Could you check a few things on this drawing? It's one solid part, dimensions in mm from its lowest x, y, z. Give positions to 0.01 mm unless a question says otherwise; leave off trailing zeros. Order: outer loops, then holes, each group sorted by start corner. A loop starts at its lowest first (then second) coordinate and runs counter-clockwise, first axis right, second up. Notation, with made-up numbers: M 11.5,-20.75 L 60.5,-20.75 A24 ccw 60.5,-6.75 Z; hole C 62,54.25 d2. An arc over 180 degrees is marked long. One line per item, written item: value. Start each with the question number.
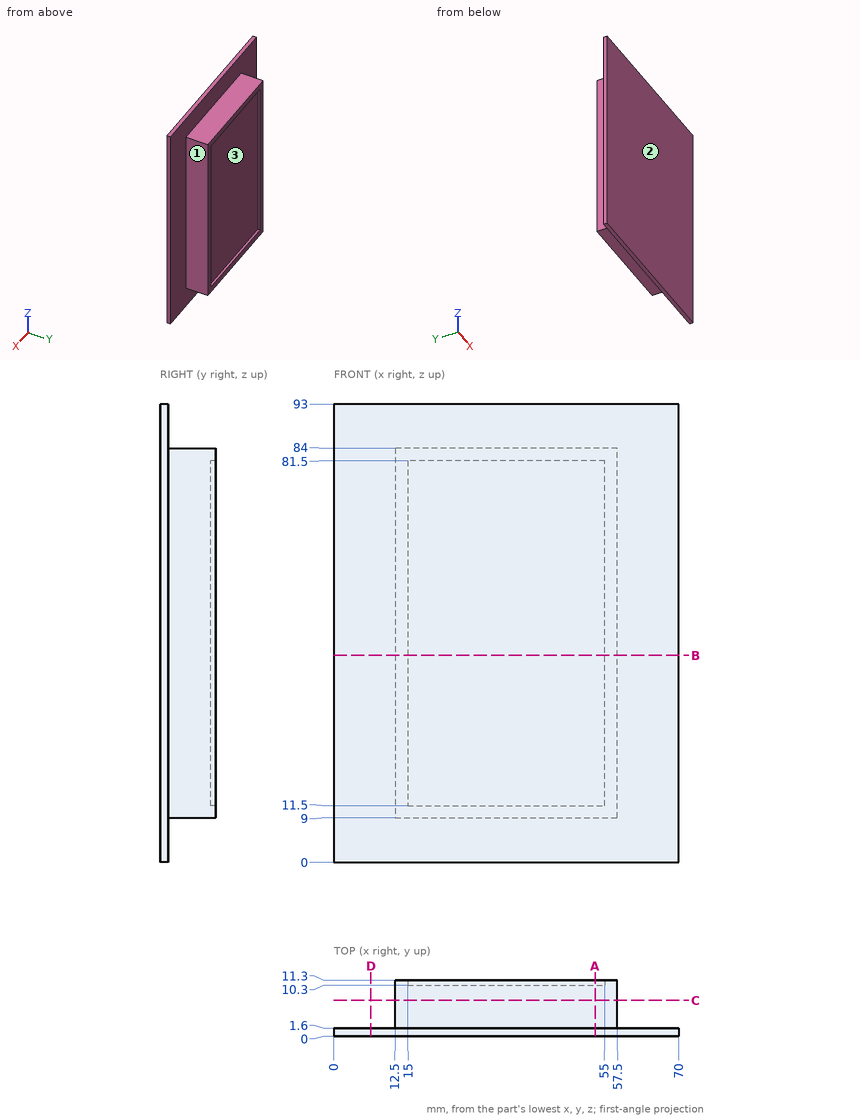
Item 1: I want a section at C-C on y = 7.25. Write out the boundary of the cut face in (x, z), plus the area to 4 significant figures.
Item 2: I want a section at D-D on x = 7.5. Write out the boundary of the cut face in (y, z).
Item 3: We'd pull the mould along X, two halves only. Please class the marked faces 1, 2 and 3: +X half, -X half, draft (parallel to the pull), parting line (faces both ways), or undercut.
Item 4: Please list where these lines run through material, in increasing order: probe 1 along Z at (x, y) = (21, 2.25); probe 2 along Y at (x, z) = (26, 25); probe 3 along X at (y, z) = (3, 36). Write a range as [from, to].
Item 5: I want a section at A-A on x = 53. Write out the boundary of the cut face in (y, z).
Item 6: Will these pins go through, and if not, where does the flat tip stop? P1, Ø20, axis at x = 40, z = 33, coming from the +Y side; P2, Ø4, axis at x = 37.5, y = 4, coming from the +Z side; P3, Ø1.1, axis at y = 10.5, z = 51.5, coming from the -X side; P4, Ø1.5, axis at x = 60, z = 18, coming from the -Y side.
Item 7: I want a section at B-B on z = 42. Write out the boundary of the cut face in (x, y).
Answer below:
1. outline: M 12.5,9 L 57.5,9 L 57.5,84 L 12.5,84 Z
1. area: 3,375 mm²
2. outline: M 0,0 L 1.6,0 L 1.6,93 L 0,93 Z
3. face 1: +X half
3. face 2: draft
3. face 3: undercut
4. probe 1: z = [9, 84]
4. probe 2: y = [0, 10.3]
4. probe 3: x = [12.5, 57.5]
5. outline: M 0,0 L 1.6,0 L 1.6,9 L 11.3,9 L 11.3,11.5 L 10.3,11.5 L 10.3,81.5 L 11.3,81.5 L 11.3,84 L 1.6,84 L 1.6,93 L 0,93 Z
6. P1: stops at y = 10.3
6. P2: stops at z = 84
6. P3: stops at x = 12.5
6. P4: stops at y = 0
7. outline: M 0,0 L 70,0 L 70,1.6 L 57.5,1.6 L 57.5,11.3 L 55,11.3 L 55,10.3 L 15,10.3 L 15,11.3 L 12.5,11.3 L 12.5,1.6 L 0,1.6 Z
